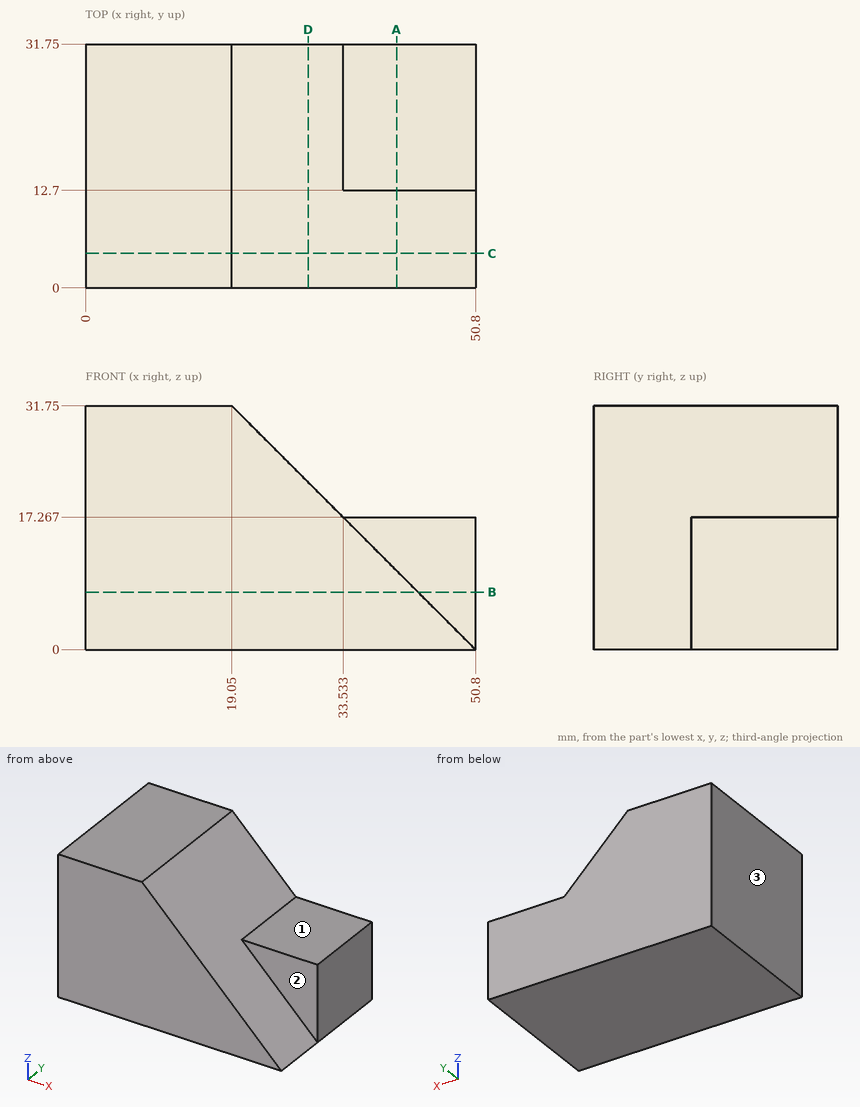
The figure shows three views and two pictorial views of one solid part (mm, origin at its lowest corner). Answer the questions. A direction names the side the tool comes from. Give positions to 0.01 mm unless a question says otherwise; leave off trailing zeros. Write each loop counter-clockwise with the first axis right and the second up, starting at its lowest first coordinate (ties: lowest second). Pieces come first, ordered by that corner, then holes. Notation, with made-up numbers: (6, -17.5) - (47, -17.5) arc R16 cw to (47, 5.5) - close; hole circle Ø7 at (45.5, 53.5). An arc over 180 degrees is marked (long way). Use CSV: the item, a comma, the result in double quotes. Start each with the question number.
Item 1: For the marked faces 1, 2 and 3, determine the directions among +Z, -Z, +X, -X, +Y, -Y from which every point of the face is accessible in a straight line to the end or side of a thin tool.
Item 2: The part is cut by section C-C, the plane y = 4.5. Give the vertices of the cut face in (x, z).
Item 3: The part is cut by section A-A, the plane x = 40.5. Give the vertices of the cut face in (y, z).
Item 4: The part is cut by section D-D, the plane x = 29. Give the vertices of the cut face in (y, z), and give its area (3 significant figures).
Item 5: Consider line 1 (Z direction, x = 45, y = 14.5); line 2 (Z direction, x = 21.5, y = 28.5); line 3 (X direction, y = 2, z = 25). Determine where each line is inside the solid, lowest interval first.
Item 6: The part is cut by section B-B, the plane z = 7.5. Give the vertices of the cut face in (x, y), and give its area (3 significant figures).
Item 7: Flat-ended cylindrical pins translate along their axes: P1, Ø10, axis at x = 29.5, y = 19.5, coming from the +Z side; P2, Ø6, axis at y = 9.5, z = 9, coming from the +X side; P3, Ø14, axis at x = 46, y = 25.5, coming from the +Z side. Find the tip coordinate at first contact, or state that the pin passes through.
Taken from the geometry:
1,face 1,"+Z, +X, +Y, -Y"
1,face 2,"+Z, +X, -Y"
1,face 3,"+Z, -Z, -X, +Y, -Y"
2,outline,"(0, 0) - (50.8, 0) - (19.05, 31.75) - (0, 31.75) - close"
3,outline,"(0, 0) - (31.75, 0) - (31.75, 17.27) - (12.7, 17.27) - (12.7, 10.3) - (0, 10.3) - close"
4,outline,"(0, 0) - (31.75, 0) - (31.75, 21.8) - (0, 21.8) - close"
4,area,"692 mm2"
5,line 1,"0 to 17.27"
5,line 2,"0 to 29.3"
5,line 3,"0 to 25.8"
6,outline,"(0, 0) - (43.3, 0) - (43.3, 12.7) - (50.8, 12.7) - (50.8, 31.75) - (0, 31.75) - close"
6,area,"1,520 mm2"
7,P1,"z = 26.3"
7,P2,"x = 44.8"
7,P3,"z = 17.27"
